Can you work these out from the model? Positions are in its coordinate system, mm. A direction names the side the tool comes from. Round coordinates to 2 decimals unless told otherwise and drop trailing zeros. Order: outer loops, then holes, each group sorted by start corner. A loop starts at its lowest first (then second) coordinate and runs counter-clockwise, first axis right, second up. Notation, with made-up numbers: M 62,68.25 L 70,68.25 A29 cw 70,101.25 Z; hole C 46.25,43 d2. An arc over 180 degrees is marked long. One line per question, with ' | ' between items.
```python
from build123d import *

# Parameters (mm, degrees)
BOSS_EXTRUDE1_DEPTH = 7
FILLET1_R           = 7


with BuildPart() as part:
    # Sketch1 → Boss-Extrude1 (new body)
    with BuildSketch(Plane(origin=(0, 0, 0), x_dir=(1, 0, 0), z_dir=(0, 1, 0))):
        with BuildLine():
            Line((0, 20), (0, 5))
            ThreePointArc((0, 5), (-5, 0), (0, -5))
            Line((0, -5), (0, -20))
            ThreePointArc((0, -20), (20, 0), (0, 20))
        make_face()
        with BuildLine():
            Line((1.112429773, -1.15), (-1.112429773, -1.15))
            ThreePointArc((-1.112429773, -1.15), (0, 1.6), (1.112429773, -1.15))
        make_face(mode=Mode.SUBTRACT)
    extrude(amount=BOSS_EXTRUDE1_DEPTH)

    # Fillet1
    fillet1_edges = [part.edges().sort_by_distance(p)[0] for p in [
        (0, 3.5, 20),
        (0, 3.5, -20),
    ]]
    fillet(fillet1_edges, radius=FILLET1_R)


solid = part.part
```
(1) Please list where these lines run through material, in increasing order: probe 1 along X at (y, z) = (2, 0); probe 2 along Z at (x, y) = (13.75, 5.5); probe 3 along X at (y, z) = (4.5, 1). Write a range as [from, to].
Final values:
probe 1: [-5, -1.6], [1.6, 20] | probe 2: [-14.52, 14.52] | probe 3: [-4.9, -1.25], [1.25, 19.97]
(2) Will these pins go through, and if not, where does the flat tip stop? pin 1 Ø1.5 at (x, y) = (3, 1) entering from +Z; pin 2 Ø2 at (y, z) = (3.5, -4.5) entering from -X; pin 3 Ø1.8 at (y, z) = (3.5, -7.5) entering from -X.
Final values:
pin 1: z = 17.15 | pin 2: x = -3.57 | pin 3: x = 0
(3) If we section it at B-B on y = 5: Please give me the cut outline in (x, z), plus the area to 3 significant figures.
Final values:
outline: M 0,-10.95 A7 ccw 10.77,-16.85 A20 ccw 10.77,16.85 A7 ccw 0,10.95 L 0,5 A5 ccw 0,-5 Z; hole M -1.11,1.15 A1.6 ccw long 1.11,1.15 Z | area: 614 mm^2
(4) If we section it at A-A on z = 0: Please give me the cut outline in (x, y), plus the area to 3 significant figures.
Final values:
outline: M -5,0 L -1.6,0 L -1.6,7 L -5,7 Z; M 1.6,0 L 20,0 L 20,7 L 1.6,7 Z | area: 153 mm^2
(5) Thinking about a two-plate mould opening in Z: for faces 3 (the flat face through (0, 3, -8)), 4 (the cylindrical face through (3.546, 3.549, -17.043)), 5 (the flat face through (0, 3, 1.15)), which applies, released by +Z, released by -Z, zero draft, split by the parting line, or undercut?
Final values:
face 3: zero draft | face 4: released by -Z | face 5: undercut
(6) On a 3-axis mill with a long thin cutter (end or side, diameter ignored), from which of +Z, -Z, +X, -X, +Y, -Y can I reach the whole of each face in a straight line? I mean faces 1 (the flat face through (7, 7, 0)), 2 (the flat face through (0, 3, 8)). Say none if no direction works.
Final values:
face 1: +Z, -Z, +X, -X, +Y | face 2: +Z, -X, +Y, -Y
(7) If we section it at D-D on z = 7: Please give me the cut outline in (x, y) (3 decimals), plus the area to 3 significant figures.
Final values:
outline: M 0,0 L 18.735,0 L 18.735,7 L 0,7 Z | area: 131 mm^2
(8) If we section it at C-C on x = 10: Please give me the cut outline in (y, z).
Final values:
outline: M 0,-17.28 L 7,-17.28 L 7,17.28 L 0,17.28 Z
